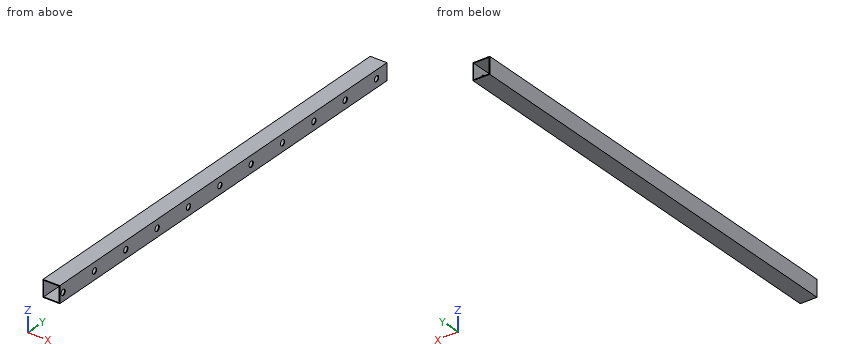
Autodesk Inventor part; units mm, degrees
ref_plane "YZ Plane" through (0, 0, 0) normal (1, 0, 0) x (0, 1, 0)
ref_plane "XZ Plane" through (0, 0, 0) normal (0, 1, 0) x (-1, 0, 0)
ref_plane "XY Plane" through (0, 0, 0) normal (0, 0, 1) x (1, 0, 0)
sketch "Sketch9" plane through (0, 0, 0) normal (0, 1, 0) x (-1, 0, 0)
  line L0 (25, 25) -> (-25, 25)
  line L1 (-25, 25) -> (-25, -25)
  line L2 (-25, -25) -> (25, -25)
  line L3 (25, -25) -> (25, 25)
  line L4 (25, 25) -> (-25, -25) construction
  line L5 (-25, 25) -> (25, -25) construction
  line L6 (-23, 23) -> (23, 23)
  line L7 (23, 23) -> (23, -23)
  line L8 (23, -23) -> (-23, -23)
  line L9 (-23, -23) -> (-23, 23)
  point P0 (0, 0)
  dimension "d172" = 50
  dimension "d173" = 50
  dimension "d174" = 2
extrude "Extrusion3" add sketch "Sketch9" against normal blind 1305
sketch "Sketch10" plane through (0, 0, 0) normal (1, 0, 0) x (0, 1, 0)
  line L0 (0, 25) -> (0, -25) construction
  line L1 (0, 25) -> (-1305, 25) construction
  line L2 (-1305, -25) -> (-1305, 25) construction
  line L3 (0, -25) -> (-1305, -25) construction
  line L4 (-1300, 8.5) -> (-1283, 8.5)
  line L5 (-1283, 8.5) -> (-1283, -8.5)
  line L6 (-1283, -8.5) -> (-1300, -8.5)
  line L7 (-1300, -8.5) -> (-1300, 8.5)
  line L8 (-1300, 8.5) -> (-1283, -8.5) construction
  line L9 (-1283, 8.5) -> (-1300, -8.5) construction
  circle A0 centre (-1291.5, 0) radius 8.5
  line L10 (0, 25) -> (0, -25)
  point P0 (0, 0)
  point P1 (0, 0)
  point P2 (-1305, 0)
  dimension "d177" = 17
  dimension "d178" = 17
  dimension "d191" = 5
extrude "Extrusion4" cut sketch "Sketch10" along normal through all contours A0
pattern_linear "Rectangular Pattern4" count 11 spacing 125 along (0, 1, 0) of "Extrusion4"
properties part number "TKS 3532 FDS WAY tube2" material "Stainless Steel"
Read the model definition and answer for the solid it produces. Units are mm, in the model's axes. Round coordinates to 2 decimals unless told otherwise and drop trailing zeros. Order: outer loops, then holes, each group sorted by start corner. A loop starts at its lowest first (then second) coordinate and runs counter-clockwise, first axis right, second up.
1) The part is cut by section B-B on z = 0. Give the number of separate pieces and of enclosed holes in the cut face, plus the area to 3 significant figures.
2) A flat-ended cylindrical pin translates along its axis: pin 1 (10 mm diameter, centred on y = -1041.5, z = 0, fed in from +X). Find the tip coordinate at first contact, or state that the pin passes through.
3) The part is cut by section A-A on y = -881. Write down the section's boundary in (x, z), plus the area to 3 significant figures.
4) Straight lines are drawn through the part: L1, parallel to X at y = -1188, z = -21.5; L2, parallel to Z at x = 24.3, y = -41.5. For each, find the intervals that lie inside material, in ascending order.
Resolved:
1. separate pieces: 13
1. enclosed holes: 0
1. area: 4,850 mm2
2. pin 1: stops at x = -23
3. outline: (-25, -25) - (25, -25) - (25, 25) - (-25, 25) - close; hole (-23, -23) - (23, -23) - (23, 23) - (-23, 23) - close
3. area: 384 mm2
4. L1: x = -25 to -23, 23 to 25
4. L2: z = -25 to -8.5, 8.5 to 25
